Input: part model. Units: mm. Frame: model coordinates. Face numbers are marked on the shaded views. A direction names the side the tool comes from. Round coordinates to 2 decimals unless told otherwise and drop trailing zeros. Order: outer loops, then holes, each group sorted by start corner. A loop starts at its lowest first (then second) coordinate and runs counter-clockwise, first axis right, second up. Notation, with made-up numbers: M -27,58 L 14,58 A21 cw 14,82 Z; hole C 12,19 d6. An arc over 180 degrees is marked long. One line per question, with ' | ' between items.
```python
from build123d import *

# Parameters (mm, degrees)
F0_R     = 4.1148
F1_DEPTH = 12.7
F2_R     = 2.54
F5_DEPTH = 4.7498


# Not quite as in the source:
# - two fillets or chamfers of one size are made in one step
# - a feature of the source that left no trace in its solid (it failed there, or was rolled back) is left out
# - a feature names something its author has since deleted; it is built from what else it names


with BuildPart() as f1:
    # F0 (on Front) → F1 (new body)
    with BuildSketch(Plane.XZ):
        Polygon((27.9026240856, 20.8031311891), (6.35, 0), (57.15, 0), (36.2365272497, 21.6669410203), (42.6968688109, 27.9026240856), (63.5, 6.35), (63.5, 57.15), (41.8330589797, 36.2365272497), (35.5973759144, 42.6968688109), (57.15, 63.5), (6.35, 63.5), (27.2634727503, 41.8330589797), (20.8031311891, 35.5973759144), (0, 57.15), (0, 6.35), (21.6669410203, 27.2634727503), align=None)
        with Locations((31.75, 31.75)):
            Circle(F0_R, mode=Mode.SUBTRACT)
    extrude(amount=F1_DEPTH)

    # F2
    f2_edges = [f1.edges().sort_by_distance(p)[0] for p in [
        (31.75, -12.7, 63.5),
        (31.75, 0, 63.5),
        (10.401566, -12.7, 46.373688),
        (63.5, -12.7, 31.75),
        (31.75, -12.7, 0),
        (31.75, 0, 0),
        (0, -12.7, 31.75),
        (16.806736, -12.7, 52.666529),
        (24.033302, -12.7, 38.715217),
        (0, -6.35, 57.15),
        (6.35, -6.35, 63.5),
        (0, 0, 31.75),
        (24.784783, 0, 24.033302),
        (24.784783, -12.7, 24.033302),
        (6.35, -6.35, 0),
        (17.126312, 0, 10.401566),
        (17.126312, -12.7, 10.401566),
        (57.15, -6.35, 0),
        (46.693264, 0, 10.833471),
        (46.693264, -12.7, 10.833471),
        (39.466698, 0, 24.784783),
        (39.466698, -12.7, 24.784783),
        (63.5, -6.35, 6.35),
        (53.098434, 0, 17.126312),
        (53.098434, -12.7, 17.126312),
        (63.5, -6.35, 57.15),
        (63.5, 0, 31.75),
        (52.666529, 0, 46.693264),
        (52.666529, -12.7, 46.693264),
        (38.715217, 0, 39.466698),
        (38.715217, -12.7, 39.466698),
        (57.15, -6.35, 63.5),
        (46.373688, 0, 53.098434),
        (46.373688, -12.7, 53.098434),
        (16.806736, 0, 52.666529),
        (24.033302, 0, 38.715217),
        (10.401566, 0, 46.373688),
        (0, -6.35, 6.35),
        (10.833471, 0, 16.806736),
        (10.833471, -12.7, 16.806736),
    ]]
    fillet(f2_edges, radius=F2_R)

    # F4 (on face) → F5 (cut)
    with BuildSketch(Plane.XZ.offset(12.7)):
        Polygon((31.75, 25.5715837887), (37.9284162113, 31.75), (31.75, 37.9284162113), (25.5715837887, 31.75), align=None)
    extrude(amount=-F5_DEPTH, mode=Mode.SUBTRACT)


solid = f1.part
```
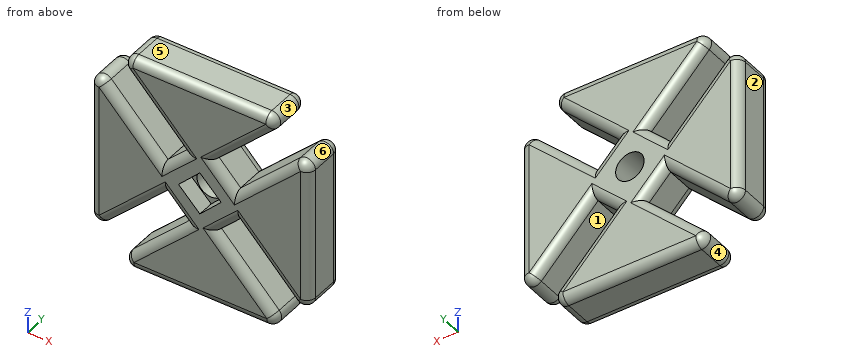
Item 1: Access query for the marked faces 1 and 2. Directions: +Z, -Z, +X, -X, +Y, -Y. A direction counts if a zero-diameter tool reaches every point of the face in a straight line with its end or side. Return the directions, or none.
Report:
face 1: +Y, -Y | face 2: +Z, -Z, -X, +Y, -Y
Item 2: Section query A-A, the plane y = -7. Return loops of the section in (x, z), plus the area to 3 significant figures.
Report:
outline: M 0,12.33 A2.54 ccw 4.3,10.5 L 21.67,27.26 L 27.9,20.8 L 10.87,4.37 A2.54 ccw 12.64,0 L 51.17,0 A2.54 ccw 53,4.3 L 36.24,21.67 L 42.7,27.9 L 59.13,10.87 A2.54 ccw 63.5,12.64 L 63.5,51.17 A2.54 ccw 59.2,53 L 41.83,36.24 L 35.6,42.7 L 52.63,59.13 A2.54 ccw 50.86,63.5 L 12.33,63.5 A2.54 ccw 10.5,59.2 L 27.26,41.83 L 20.8,35.6 L 4.37,52.63 A2.54 ccw 0,50.86 Z; hole C 31.75,31.75 d8.23 | area: 2,760 mm²
Item 3: Section query B-B, the plane x = 44. Give the number of separate pieces and of enclosed holes in the cut face, plus the area to 3 significant figures.
Report:
separate pieces: 3 | enclosed holes: 0 | area: 463 mm²
Item 4: First-contact query: pin 1 (6 mm diameter, centred on x = 56.5, y = -8.5, fed in from -Z); pin 2 (2 mm diameter, centred on y = -10.5, z = 7, fed in from -X); pin 3 (6 mm diameter, centred on x = 9.5, y = -7, fed in from -Z). Flat tips, straight axial feed; report the tip coordinate or a pass-through.
Report:
pin 1: z = 1.53 | pin 2: x = 12.59 | pin 3: z = 0
Item 5: Mould query, pull axis X, two halves, no side actions, for the marked faces 3, 4, 5 and 6. Classes: +X half, -X half, draft (parallel to the pull), parting line (faces both ways), or undercut.
Report:
face 3: +X half | face 4: -X half | face 5: draft | face 6: undercut
Item 6: Section query C-C, the plane y = -1.75. Return loops of the section in (x, z).
Report:
outline: M 0.13,12.33 A2.41 ccw 4.22,10.59 L 21.67,27.44 L 28.08,20.8 L 10.96,4.28 A2.41 ccw 12.64,0.13 L 51.17,0.13 A2.41 ccw 52.91,4.22 L 36.06,21.67 L 42.7,28.08 L 59.22,10.96 A2.41 ccw 63.37,12.64 L 63.37,51.17 A2.41 ccw 59.28,52.91 L 41.83,36.06 L 35.42,42.7 L 52.54,59.22 A2.41 ccw 50.86,63.37 L 12.33,63.37 A2.41 ccw 10.59,59.28 L 27.44,41.83 L 20.8,35.42 L 4.28,52.54 A2.41 ccw 0.13,50.86 Z; hole C 31.75,31.75 d8.23
Item 7: Line query: line 1 along X through (y, z) = (-3, 31.75); line 2 along Z through (x, y) = (12, -3.75); line 3 along X through (y, z) = (-10.25, 42). Output: solid intervals per line, ascending. Write a range as from..to.
Report:
line 1: 0..27.64, 35.86..63.5 | line 2: 0.08..5.45, 17.93..44.72, 57.65..63.48 | line 3: 0..14.62, 27.1..36.27, 47.81..63.5
